Can you work these out from the model? Positions are in its coordinate system, mm. A direction names the side the tool comes from. Give positions to 0.01 mm unless a question says otherwise; leave off trailing zeros. Order: outer loops, then holes, each group sorted by start corner. A loop starts at its lowest first (then second) coordinate and runs counter-clockwise, first axis right, second up. Notation, with made-up numbers: (35.5, 7.5) - (85.5, 7.5) arc R23 cw to (85.5, 41.5) - close; hole circle Ø3 at (21, 85). An arc over 180 degrees is marked (long way). Return JSON: item names as keys, results as strings.
```python
from build123d import *

# Parameters (mm, degrees)
EXTRUDE_THIN1_DEPTH = 20.6375
SKETCH2_R           = 7.14375
CUT_EXTRUDE1_DEPTH  = 533.454292692
SKETCH3_R           = 7.14375
CUT_EXTRUDE2_DEPTH  = 533.454292692


with BuildPart() as part:
    # Sketch1 → Extrude-Thin1 (new, symmetric)
    with BuildSketch(Plane.XY):
        Polygon((-256.801146906, -215.526146906), (-215.526146906, -215.526146906), (215.526146906, 215.526146906), (215.526146906, 256.801146906), (209.176146906, 256.801146906), (209.176146906, 218.156403027), (-218.156403027, -209.176146906), (-256.801146906, -209.176146906), align=None)
    extrude(amount=EXTRUDE_THIN1_DEPTH, both=True)

    # Sketch2 → Cut-Extrude1 (cut, through all)
    with BuildSketch(Plane(origin=(0, -209.176146906, 0), x_dir=(1, 0, 0), z_dir=(0, 1, 0))):
        with Locations(Location((-236.163646906, 0, 0), (0, 0, 270))):
            Circle(SKETCH2_R)
    extrude(amount=-CUT_EXTRUDE1_DEPTH, mode=Mode.SUBTRACT)

    # Sketch3 → Cut-Extrude2 (cut, through all)
    with BuildSketch(Plane.ZY.offset(-209.176146906)):
        with Locations(Location((0, 236.163646906, 0), (0, 0, 270))):
            Circle(SKETCH3_R)
    extrude(amount=-CUT_EXTRUDE2_DEPTH, mode=Mode.SUBTRACT)


solid = part.part
```
1. On a 3-axis mill with a long thin cutter (end or side, diameter ignored), from which of +Z, -Z, +X, -X, +Y, -Y can I reach the whole of each face in a straight line? I mean faces 1 (the face through (215.526, 227, 0)), 2 (the face through (-242, -209.176, 5)). Say none if no direction works.
Checks:
{"face 1": "+Z, -Z, +X, +Y, -Y", "face 2": "+Z, -Z, -X, +Y"}
2. If I drill on L1, parallel to X at y = 227, z = 13.5; L2, parallel to Y at x = -229, z = 11.5; L3, parallel to X at y = -211, z = 0, over which ranges is the centre line in solid material (lowest first)? Write a range as [from, to].
Checks:
{"L1": "[209.18, 215.53]", "L2": "[-215.53, -209.18]", "L3": "[-256.8, -243.31], [-229.02, -211]"}
3. Suppose I cut it at A-A (z = 0). List the corners of the cut face in (x, y) for me.
Checks:
{"outline": "(-256.8, -215.53) - (-243.31, -215.53) - (-243.31, -209.18) - (-256.8, -209.18) - close; (-229.02, -215.53) - (-215.53, -215.53) - (215.53, 215.53) - (215.53, 229.02) - (209.18, 229.02) - (209.18, 218.16) - (-218.16, -209.18) - (-229.02, -209.18) - close; (209.18, 243.31) - (215.53, 243.31) - (215.53, 256.8) - (209.18, 256.8) - close"}
4. Thinking about a two-plate mould opening in Z: for faces 3 (the face through (-240.51, -212.31, -5.67)), 4 (the face through (-1.5, 7.48, 0.29)), 5 (the face through (-4, 4, -20.638)), which applies, +Z half, -Z half, draft (parallel to the pull), parting line (faces both ways), or undercut?
Checks:
{"face 3": "undercut", "face 4": "draft", "face 5": "-Z half"}
5. For pin 1 Ø8 at (y, z) = (7, -4.5) entering from -X; pin 2 Ø11.5 at (y, z) = (239.5, -6.5) entering from -X; pin 3 Ø13 at (y, z) = (236.16, 0) entering from +X; pin 4 Ø10 at (y, z) = (-75, 0) entering from +X, each with a flat end and sliding along its axis, tell me the tip position at first contact or that it passes through.
Checks:
{"pin 1": "x = -5.98", "pin 2": "x = 209.18", "pin 3": "through", "pin 4": "x = -70"}
6. Suppose I cut it at C-C (y = 117). List the corners of the cut face in (x, z) for me, plus the area to 3 significant figures.
Checks:
{"outline": "(108.02, -20.64) - (117, -20.64) - (117, 20.64) - (108.02, 20.64) - close", "area": "371 mm^2"}
7. Suppose I cut it at B-B (x = -17). List the corners of the cut face in (y, z) for me.
Checks:
{"outline": "(-17, -20.64) - (-8.02, -20.64) - (-8.02, 20.64) - (-17, 20.64) - close"}
